Source: CAD feature listing. Evaluate the final solid. Frame: model axes, mm. A direction names the side the tool comes from. Give positions to 0.01 mm unless a question says otherwise; leave off trailing zeros. Order: outer loops, then holes, each group sorted by start corner. A loop starts at its lowest first (then second) coordinate and runs counter-clockwise, first axis right, second up. Notation, with made-up numbers: M 45,17.25 L 98,17.25 A7 ccw 98,24.25 Z; hole C 28,53.25 d4. An arc over 180 degrees is marked long. Return JSON: item names as keys, results as strings.
from build123d import *

# Parameters (mm, degrees)
SALIENTE_EXTRUIR1_DEPTH  = 10
CROQUIS2_W               = 5
CROQUIS2_H               = 45
CORTAR_EXTRUIR1_DEPTH    = 12.5
CROQUIS4_W               = 73.322426794
CROQUIS4_H               = 5
SALIENTE_EXTRUIR2_DEPTH  = 30
CROQUIS5_W               = 2.5
CROQUIS5_H               = 5
SALIENTE_EXTRUIR3_DEPTH  = 50
CROQUIS6_W               = 55.637494131
CROQUIS6_H               = 64.414873678
CORTAR_EXTRUIR2_DEPTH    = 55
CROQUIS7_R               = 1.5
CORTAR_EXTRUIR3_DEPTH    = 5
CROQUIS8_W               = 39.981329184
CROQUIS8_H               = 5
CORTAR_EXTRUIR4_DEPTH    = 10
CROQUIS9_W               = 10
CROQUIS9_H               = 7.5
SALIENTE_EXTRUIR4_DEPTH  = 21
CROQUIS11_R              = 2
CORTAR_EXTRUIR5_DEPTH    = 21
SALIENTE_EXTRUIR5_START  = -40
CROQUIS12_W              = 21.008716652
CROQUIS12_H              = 5
SALIENTE_EXTRUIR5_DEPTH  = 40
CORTAR_EXTRUIR6_DEPTH    = 62.200166864
CROQUIS15_W              = 5
CROQUIS15_H              = 10
SALIENTE_EXTRUIR6_DEPTH  = 31.1
SALIENTE_EXTRUIR7_DEPTH  = 10
SALIENTE_EXTRUIR8_DEPTH  = 5
CORTAR_EXTRUIR7_START    = -13
CROQUIS21_R              = 1.5
CORTAR_EXTRUIR7_DEPTH    = 13
CROQUIS22_W              = 10
CROQUIS22_H              = 7.5
CORTAR_EXTRUIR14_DEPTH   = 75.112484941
CROQUIS26_W              = 65
CROQUIS26_H              = 5
SALIENTE_EXTRUIR11_DEPTH = 10
SALIENTE_EXTRUIR12_DEPTH = 5
CORTAR_EXTRUIR15_START   = -10
CROQUIS28_R              = 1.5
CORTAR_EXTRUIR15_DEPTH   = 10
CROQUIS29_W              = 10
CROQUIS29_H              = 16.1
SALIENTE_EXTRUIR13_DEPTH = 5


with BuildPart() as part:
    # Croquis1 → Saliente-Extruir1 (new body)
    with BuildSketch(Plane.XY):
        with BuildLine():
            Line((-35, 10), (-35, 0))
            Line((-35, 0), (-30, 0))
            Line((-30, 0), (-30, 10))
            Line((-30, 10), (-20, 10))
            Line((-20, 10), (-20, 35.723707224))
            ThreePointArc((-20, 35.723707224), (0, 55.723707224), (20, 35.723707224))
            Line((20, 35.723707224), (20, 10))
            Line((20, 10), (30, 10))
            Line((30, 10), (30, 0))
            Line((30, 0), (35, 0))
            Line((35, 0), (35, 10))
            Line((35, 10), (39, 10))
            Line((39, 10), (39, 20))
            Line((39, 20), (14.443351433, 84.048407017))
            Line((14.443351433, 84.048407017), (13.447706691, 86.645237749))
            ThreePointArc((13.447706691, 86.645237749), (0, 95), (-13.447706691, 86.645237749))
            Line((-13.447706691, 86.645237749), (-14.443351433, 84.048407017))
            Line((-14.443351433, 84.048407017), (-39, 20))
            Line((-39, 20), (-39, 10))
            Line((-39, 10), (-35, 10))
        make_face()
        with BuildLine():
            ThreePointArc((1.5, 60), (0, 58.5), (-1.5, 60))
            Line((-1.5, 60), (-1.5, 80))
            ThreePointArc((-1.5, 80), (0, 81.5), (1.5, 80))
            Line((1.5, 80), (1.5, 60))
        make_face(mode=Mode.SUBTRACT)
    extrude(amount=SALIENTE_EXTRUIR1_DEPTH)

    # Croquis2 → Cortar-Extruir1 (cut, symmetric)
    with BuildSketch(Plane(origin=(0, 0, 0), x_dir=(0, 0, -1), z_dir=(1, 0, 0))):
        with Locations((-5, 72.5)):
            Rectangle(CROQUIS2_W, CROQUIS2_H)
    extrude(amount=CORTAR_EXTRUIR1_DEPTH, both=True, mode=Mode.SUBTRACT)

    # Croquis4 → Saliente-Extruir2 (add)
    with BuildSketch(Plane(origin=(0, 0, 0), x_dir=(-1, 0, 0), z_dir=(0, 0, -1))):
        with Locations((0, 28.6)):
            Rectangle(CROQUIS4_W, CROQUIS4_H)
    extrude(amount=SALIENTE_EXTRUIR2_DEPTH)

    # Croquis5 → Saliente-Extruir3 (add)
    with BuildSketch(Plane(origin=(-20, 0, 0), x_dir=(0, 0, -1), z_dir=(1, 0, 0))):
        with Locations((-8.75, 28.6)):
            Rectangle(CROQUIS5_W, CROQUIS5_H)
    extrude(amount=SALIENTE_EXTRUIR3_DEPTH)

    # Croquis6 → Cortar-Extruir2 (cut, symmetric)
    with BuildSketch(Plane(origin=(-20, 0, 0), x_dir=(0, 0, -1), z_dir=(1, 0, 0))):
        with Locations((17.818747066, 63.307436839)):
            Rectangle(CROQUIS6_W, CROQUIS6_H)
    extrude(amount=CORTAR_EXTRUIR2_DEPTH, both=True, mode=Mode.SUBTRACT)

    # Croquis7 → Cortar-Extruir3 (cut)
    with BuildSketch(Plane.XY.offset(10)):
        with Locations((0, 28.6)):
            Circle(CROQUIS7_R)
    extrude(amount=-CORTAR_EXTRUIR3_DEPTH, mode=Mode.SUBTRACT)

    # Croquis8 → Cortar-Extruir4 (cut)
    with BuildSketch(Plane(origin=(0, 31.1, 0), x_dir=(1, 0, 0), z_dir=(0, 1, 0))):
        with Locations((-0.009335408, 2.5)):
            Rectangle(CROQUIS8_W, CROQUIS8_H)
    extrude(amount=-CORTAR_EXTRUIR4_DEPTH, mode=Mode.SUBTRACT)

    # Croquis9 → Saliente-Extruir4 (add)
    with BuildSketch(Plane(origin=(0, 31.1, 0), x_dir=(1, 0, 0), z_dir=(0, 1, 0))):
        with Locations((15.061213397, 24.25)):
            Rectangle(CROQUIS9_W, CROQUIS9_H)
        with Locations((-35.940317185, 24.25)):
            Rectangle(CROQUIS9_W, CROQUIS9_H)
    extrude(amount=SALIENTE_EXTRUIR4_DEPTH)

    # Croquis11 → Cortar-Extruir5 (cut)
    with BuildSketch(Plane.XY.offset(-20.5)):
        with Locations((13.560448106, 46.6)):
            Circle(CROQUIS11_R)
        with Locations((13.560448106, 35.6)):
            Circle(CROQUIS11_R)
        with Locations((-34.439551894, 46.6)):
            Circle(CROQUIS11_R)
        with Locations((-34.439551894, 35.6)):
            Circle(CROQUIS11_R)
    extrude(amount=-CORTAR_EXTRUIR5_DEPTH, mode=Mode.SUBTRACT)

    # Croquis12 → Saliente-Extruir5 (add)
    with BuildSketch(Plane(origin=(0, 0, -30), x_dir=(-1, 0, 0), z_dir=(0, 0, -1)).offset(SALIENTE_EXTRUIR5_START)):
        with Locations((32.834428277, 28.6)):
            Rectangle(CROQUIS12_W, CROQUIS12_H)
    extrude(amount=SALIENTE_EXTRUIR5_DEPTH)

    # Croquis13 → Cortar-Extruir6 (cut, through all)
    with BuildSketch(Plane(origin=(0, 31.1, 0), x_dir=(1, 0, 0), z_dir=(0, 1, 0))):
        Polygon((34.744175198, 0), (36.661213397, 0), (36.661213397, 30), (21.661213397, 30), align=None)
    extrude(amount=-CORTAR_EXTRUIR6_DEPTH, mode=Mode.SUBTRACT)

    # Croquis15 → Saliente-Extruir6 (add)
    with BuildSketch(Plane(origin=(0, 31.1, 0), x_dir=(1, 0, 0), z_dir=(0, 1, 0))):
        with Locations((0, 25)):
            Rectangle(CROQUIS15_W, CROQUIS15_H)
    extrude(amount=-SALIENTE_EXTRUIR6_DEPTH)

    # Croquis18 → Saliente-Extruir7 (add)
    with BuildSketch(Plane.XY.offset(10)):
        Polygon((-39, 10), (-43.338786603, 26.1), (-36.661213397, 26.1), align=None)
    extrude(amount=-SALIENTE_EXTRUIR7_DEPTH)

    # Croquis22 → Cortar-Extruir14 (cut, through all)
    with BuildSketch(Plane(origin=(0, 52.1, 0), x_dir=(1, 0, 0), z_dir=(0, 1, 0))):
        with Locations((-35.940317185, 24.25)):
            Rectangle(CROQUIS22_W, CROQUIS22_H)
        with Locations((15.061213397, 24.25)):
            Rectangle(CROQUIS22_W, CROQUIS22_H)
    extrude(amount=-CORTAR_EXTRUIR14_DEPTH, mode=Mode.SUBTRACT)

    # Croquis26 → Saliente-Extruir11 (add)
    with BuildSketch(Plane(origin=(0, 0, -30), x_dir=(-1, 0, 0), z_dir=(0, 0, -1))):
        with Locations((10.838786603, 28.6)):
            Rectangle(CROQUIS26_W, CROQUIS26_H)
    extrude(amount=SALIENTE_EXTRUIR11_DEPTH)



with BuildPart() as body_2:
    # Croquis20 → Saliente-Extruir8 (new body)
    with BuildSketch(Plane(origin=(0, 31.1, 0), x_dir=(1, 0, 0), z_dir=(0, 1, 0))):
        Polygon((-1.624735856, -15), (1.624735856, -15), (34.744175198, -10), (-43.338786603, -10), align=None)
    extrude(amount=-SALIENTE_EXTRUIR8_DEPTH)

    # Croquis21 → Cortar-Extruir7 (cut)
    with BuildSketch(Plane(origin=(0, 0, 7.5), x_dir=(-1, 0, 0), z_dir=(0, 0, -1)).offset(CORTAR_EXTRUIR7_START)):
        with Locations((0, 28.6)):
            Circle(CROQUIS21_R)
    extrude(amount=CORTAR_EXTRUIR7_DEPTH, mode=Mode.SUBTRACT)


with BuildPart() as part_1:
    add(part.part)

    add(body_2.part)  # Saliente-Extruir12 merges body 2
    # Croquis27 → Saliente-Extruir12 (add)
    with BuildSketch(Plane(origin=(0, 31.1, 0), x_dir=(1, 0, 0), z_dir=(0, 1, 0))):
        Polygon((-43.338786603, -10), (-43.338786603, -8.609959484), (34.744175198, -8.609959484), (34.744175198, -10), (1.624735856, -15), (-1.624735856, -15), align=None)
    extrude(amount=-SALIENTE_EXTRUIR12_DEPTH)

    # Croquis28 → Cortar-Extruir15 (cut)
    with BuildSketch(Plane(origin=(0, 0, 8.609959484), x_dir=(-1, 0, 0), z_dir=(0, 0, -1)).offset(CORTAR_EXTRUIR15_START)):
        with Locations(Location((0, 28.6, 0), (0, 0, 180))):
            Circle(CROQUIS28_R)
    extrude(amount=CORTAR_EXTRUIR15_DEPTH, mode=Mode.SUBTRACT)

    # Croquis29 → Saliente-Extruir13 (add, symmetric)
    with BuildSketch(Plane.ZY):
        with Locations((-25, 18.05)):
            Rectangle(CROQUIS29_W, CROQUIS29_H)
    extrude(amount=SALIENTE_EXTRUIR13_DEPTH, both=True)


solid = part_1.part
1. Section query C-C (x = -13). Return loops of the section in (y, z).
Evaluation:
{"outline": "M 26.1,-40 L 31.1,-40 L 31.1,-5 L 26.1,-5 Z; M 26.1,7.5 L 31.1,7.5 L 31.1,13.64 L 26.1,13.64 Z"}
2. Section query B-B (x = 0). Return loops of the section in (y, z).
Evaluation:
{"outline": "M 0,-30 L 26.1,-30 L 26.1,-40 L 31.1,-40 L 31.1,-5 L 26.1,-5 L 26.1,-20 L 0,-20 Z; M 26.1,7.5 L 27.1,7.5 L 27.1,15 L 26.1,15 Z; M 30.1,7.5 L 31.1,7.5 L 31.1,15 L 30.1,15 Z"}
3. Section query D-D (y = 28.6). State how many separate pieces and enclosed holes the cut face has, then the cut area to 3 significant figures.
Evaluation:
{"separate pieces": "1", "enclosed holes": "2", "area": "3,120 mm^2"}
4. First-contact query: pin 1 (5 mm diameter, centred on x = 0, y = 19, fed in from -Z); pin 2 (5.5 mm diameter, centred on y = 29, z = -37, fed in from +X); pin 3 (1 mm diameter, centred on x = 11.5, z = -17.5, fed in from -Y); pin 4 (1.5 mm diameter, centred on y = 25, z = -12, fed in from +X). Flat tips, straight axial feed; report the tip coordinate or a pass-through.
Evaluation:
{"pin 1": "stops at z = -30", "pin 2": "stops at x = 21.66", "pin 3": "stops at y = 26.1", "pin 4": "passes through"}
5. Draft query along X for faces 1 (the face through (36.902, 25.472, 4.93)), 2 (the face through (-30.94, 29, -24)), 3 (the face through (-43.339, 29, -15)), 4 (the face through (-40.94, 29, -24)). Return one class per face: pulls with the +X half, pulls with the -X half, needs draft (parallel to the pull), parting line crosses it, or undercut.
Evaluation:
{"face 1": "pulls with the +X half", "face 2": "undercut", "face 3": "pulls with the -X half", "face 4": "undercut"}
6. Ray query, probe 1 along X at (y, z) = (8.5, 3); probe 2 along Y at (x, z) = (0, 13); probe 3 along Z at (x, y) = (-33, 1.5). Return the intervals inside material, ascending.
Evaluation:
{"probe 1": "x = -35 to -30, 30 to 35", "probe 2": "y = 26.1 to 27.1, 30.1 to 31.1", "probe 3": "z = 0 to 10"}
7. Set-up query: faces 5 (the face through (5, 18, -25)), 6 (the face through (-0.3, 26.9, 7.5)), 7 (the face through (-35, 5, 5)), 8 (the face through (-32, 16, 10)). Return all of +Z, -Z, +X, -X, +Y, -Y with unobstructed straight access to the full face (end or side cutting, diameter ignored); none if empty.
Evaluation:
{"face 5": "+Z, -Z, +X, -Y", "face 6": "+Y, -Y", "face 7": "+Z, -Z, -X, -Y", "face 8": "+Z, +X, -X, -Y"}
8. Section query A-A (y = 7.5). Return loops of the section in (x, z).
Evaluation:
{"outline": "M -35,0 L -30,0 L -30,10 L -35,10 Z; M -2.5,-30 L 2.5,-30 L 2.5,-20 L -2.5,-20 Z; M 30,0 L 35,0 L 35,10 L 30,10 Z"}
